Build history of the part. All positions in model axes, mm. Coordinates: 2 decimals unless noted, no trailing zeros. Order: outer loops, then holes, each group sorted by start corner. A loop starts at its lowest first (then second) coordinate and runs counter-clockwise, first axis right, second up. Notation, with made-up numbers: (46, 48) - (96, 48) arc R34 cw to (96, 81) - close; hole circle Ø5 at (74.25, 83.5). An arc over 180 degrees is marked (long way). One line per item, written item: value.
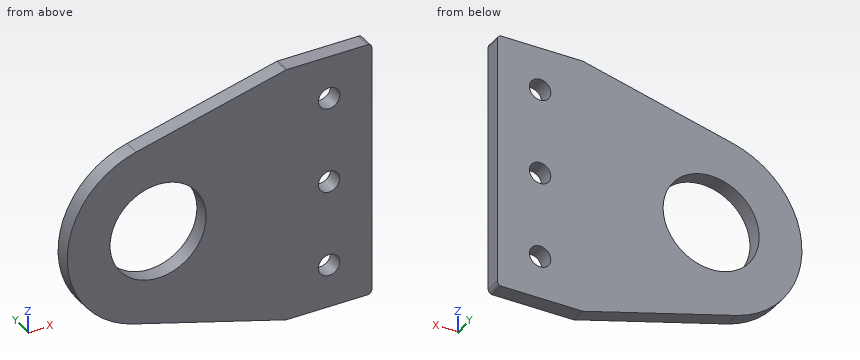
from build123d import *

# Parameters (mm, degrees)
F0_R     = 14.2748
F1_DEPTH = 4.7625
F2_D     = 6.35
F3_R     = 1.27


with BuildPart() as f1:
    # F0 (on Front) → F1 (new body)
    with BuildSketch(Plane.XZ):
        with BuildLine():
            Line((-29.2914260553, -14.6972390882), (-29.2914260553, 61.5027609118))
            Line((-29.2914260553, 61.5027609118), (-54.6914260553, 61.5027609118))
            Line((-54.6914260553, 61.5027609118), (-99.2620043736, 50.4898616483))
            ThreePointArc((-99.2620043736, 50.4898616483), (-119.7615401749, 24.805395053), (-100.2335245042, -1.6252575368))
            Line((-100.2335245042, -1.6252575368), (-54.6914260553, -14.6972390882))
            Line((-54.6914260553, -14.6972390882), (-29.2914260553, -14.6972390882))
        make_face()
        with Locations((-92.7914260553, 24.3026233199)):
            Circle(F0_R, mode=Mode.SUBTRACT)
    extrude(amount=F1_DEPTH)

    # F2 (through all)
    with Locations(Plane(origin=(0, 0, 0), x_dir=(1, 0, 0), z_dir=(0, 1, 0))):
        with Locations((-41.9914260553, -48.8027609118), (-41.9914260553, -23.4027609118), (-41.9914260553, 1.9972390882)):
            Hole(F2_D / 2)

    # F3
    f3_edges = [f1.edges().sort_by_distance(p)[0] for p in [
        (-29.291426, -2.38125, 61.502761),
        (-29.291426, -2.38125, -14.697239),
        (-54.691426, -2.38125, 61.502761),
        (-54.691426, -2.38125, -14.697239),
    ]]
    fillet(f3_edges, radius=F3_R)


solid = f1.part
1. Band-saw the part on B-B, the plane z = -3. Give the cut face in (x, y), and give its area (3 significant figures).
Values found:
outline: (-95.44, -4.76) - (-45, -4.76) - (-45, 0) - (-95.44, 0) - close; (-38.98, -4.76) - (-29.29, -4.76) - (-29.29, 0) - (-38.98, 0) - close
area: 286 mm2
2. Band-saw the part on C-C, the plane y = -2.2. Count the separate pieces of the cut face and the enclosed holes in it, and give its area (3 significant figures).
Values found:
separate pieces: 1
enclosed holes: 4
area: 4,860 mm2
3. Band-saw the part on A-A, the plane x = -94.5. Give the cut face in (y, z).
Values found:
outline: (-4.76, -3.27) - (0, -3.27) - (0, 10.13) - (-4.76, 10.13) - close; (-4.76, 38.47) - (0, 38.47) - (0, 51.67) - (-4.76, 51.67) - close
4. Flat gauge pins, fed straight in: P1, Ø1, axis at x = -62.5, y = -2.5, coming from the -Z side; P2, Ø1.5, axis at y = -2, z = 11.5, coming from the -X side. Where does each tip first touch, or does it go through?
Values found:
P1: stops at z = -12.6
P2: stops at x = -116.92
5. Band-saw the part on D-D, the plane x = -44. Give the cut face in (y, z).
Values found:
outline: (-4.76, -14.7) - (0, -14.7) - (0, -4.46) - (-4.76, -4.46) - close; (-4.76, 0.46) - (0, 0.46) - (0, 20.94) - (-4.76, 20.94) - close; (-4.76, 25.86) - (0, 25.86) - (0, 46.34) - (-4.76, 46.34) - close; (-4.76, 51.26) - (0, 51.26) - (0, 61.5) - (-4.76, 61.5) - close
6. Probe line 1 along X through (y, z) = (-4, 37); line 2 along X through (y, z) = (-1.7, 28.5); line 3 along Z through (x, y) = (-96.5, -2.3). List the from-to ranges inside material, lowest first.
Values found:
line 1: x = -116.59 to -99.31, -86.27 to -29.29
line 2: x = -119.44 to -106.44, -79.15 to -29.29
line 3: z = -2.7 to 10.52, 38.09 to 51.17
